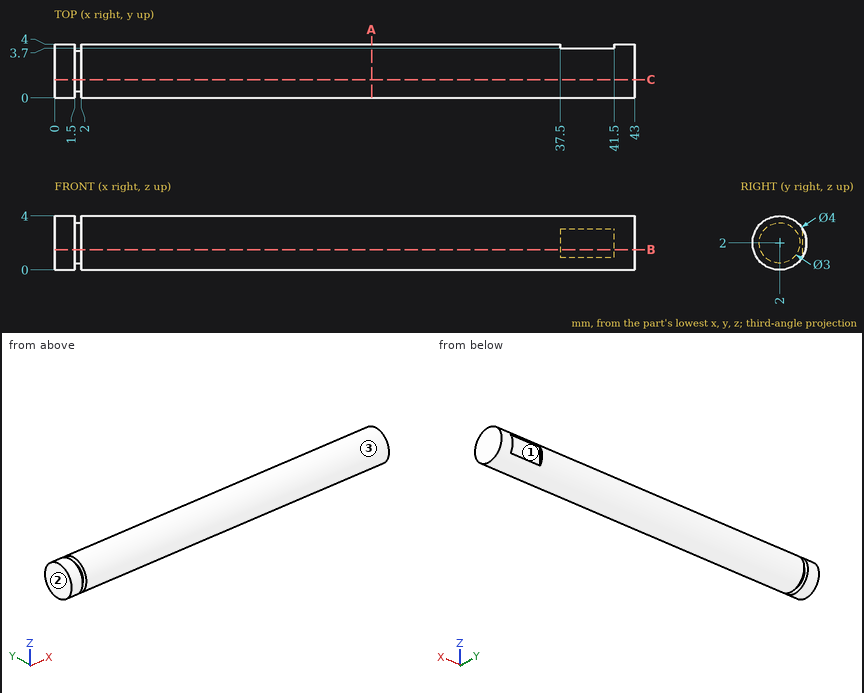
Job drawing, mm, ordinate dimensions from the low corner. One solid piece. Give positions to 0.01 mm unless a question says otherwise; leave off trailing zeros. Loops run counter-clockwise (first coordinate to the right, second up) from the corner with the lowest first, then second, coordinate; pieces in that order, holes last. Notation, with made-up numbers: M 45,72 L 74,72 A25 ccw 74,86 Z; hole C -14,-19.5 d3. An arc over 180 degrees is marked long. Answer in a Markdown table with one row per item. Add a question column.
Item 1: Probe probe 1 along X at (y, z) = (3, 0.75); probe 2 along Z at (x, y) = (29, 1.85); probe 3 along Y at (x, z) = (40, 0.9). List the from-to ranges inside material, lowest first.
Item 2: Band-saw the part on B-B on z = 1.5. Give the cut face in (x, y), then the cut area to 3 significant figures.
Item 3: Band-saw the part on C-C on y = 1.35. Give the cut face in (x, z).
Item 4: Band-saw the part on A-A on x = 23.5. Give the cut face in (y, z).
Item 5: Mould opens along X. For the marked faces 1, 2 and 3 say: +X half, -X half, draft (parallel to the pull), parting line (faces both ways), or undercut.
Item 6: Drop flat-ended pins along their axis: P1, Ø1.5, axis at y = 1, z = 3, coming from the -X side; P2, Ø1.1, axis at x = 39.5, z = 2, coming from the +Y side. Give the stop position or say it passes through.
Reply:
| question | item | result |
|---|---|---|
| 1 | probe 1 | x = 0 to 1.5, 2 to 43 |
| 1 | probe 2 | z = 0.01 to 3.99 |
| 1 | probe 3 | y = 0.33 to 3.67 |
| 2 | outline | M 0,0.06 L 1.5,0.06 L 1.5,0.59 L 2,0.59 L 2,0.06 L 43,0.06 L 43,3.94 L 41.5,3.94 L 41.5,3.7 L 37.5,3.7 L 37.5,3.94 L 2,3.94 L 2,3.41 L 1.5,3.41 L 1.5,3.94 L 0,3.94 Z |
| 2 | area | 165 mm^2 |
| 3 | outline | M 0,0.11 L 1.5,0.11 L 1.5,0.65 L 2,0.65 L 2,0.11 L 43,0.11 L 43,3.89 L 2,3.89 L 2,3.35 L 1.5,3.35 L 1.5,3.89 L 0,3.89 Z |
| 4 | outline | C 2,2 d4 |
| 5 | face 1 | undercut |
| 5 | face 2 | -X half |
| 5 | face 3 | draft |
| 6 | P1 | stops at x = 0 |
| 6 | P2 | stops at y = 3.7 |
